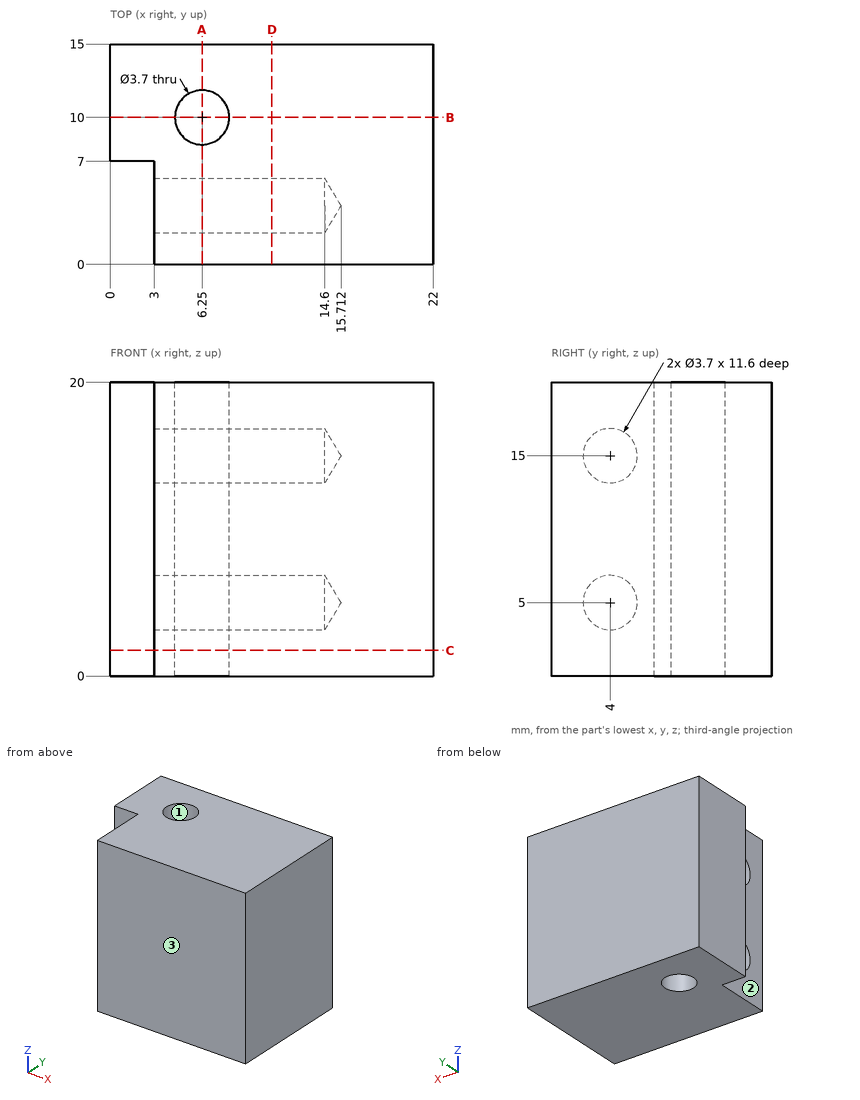
Job drawing, mm, ordinate dimensions from the low corner. One solid piece. Round coordinates to 2 decimals unless told otherwise and drop trailing zeros. Loops run counter-clockwise (first coordinate to the right, second up) from the corner with the lowest first, then second, coordinate; pieces in that order, holes last.
Item 1: Cut at D-D, the plane x = 11. Give the cut face in (y, z).
Item 2: Cut at B-B, the plane y = 10. Give the cut face in (x, z).
Item 3: Mould opens along X. For the marked faces 1, 2 and 3 say: +X half, -X half, draft (parallel to the pull), parting line (faces both ways), or undercut.
Item 4: Drill centre lines: line 1 (Z direction, x = 6.5, y = 4); line 2 (Y direction, x = 6.5, z = 15); line 3 (Y direction, x = 7, z = 14.5). Where is each one in solid material? Low to high.
Item 5: Cut at C-C, the plane z = 1.75. Give the cut face in (x, y).
Item 6: Drop flat-ended pins along their axis: P1, Ø4.5, axis at y = 4, z = 15, coming from the -X side; P2, Ø1.5, axis at x = 1, z = 10, coming from the -Y side. Give the stop position or say it passes through.
Item 7: Cut at A-A, the plane x = 6.25. Give the cut face in (y, z).
A:
1. outline: (0, 0) - (15, 0) - (15, 20) - (0, 20) - close; hole circle Ø3.7 at (4, 5); hole circle Ø3.7 at (4, 15)
2. outline: (0, 0) - (4.4, 0) - (4.4, 20) - (0, 20) - close; (8.1, 0) - (22, 0) - (22, 20) - (8.1, 20) - close
3. face 1: undercut
3. face 2: -X half
3. face 3: draft
4. line 1: z = 0 to 3.15, 6.85 to 13.15, 16.85 to 20
4. line 2: y = 0 to 2.15, 5.85 to 8.17, 11.83 to 15
4. line 3: y = 0 to 2.22, 5.78 to 8.31, 11.69 to 15
5. outline: (0, 7) - (3, 7) - (3, 0) - (22, 0) - (22, 15) - (0, 15) - close; hole circle Ø3.7 at (6.25, 10)
6. P1: stops at x = 3
6. P2: stops at y = 7
7. outline: (0, 0) - (8.15, 0) - (8.15, 20) - (0, 20) - close; (11.85, 0) - (15, 0) - (15, 20) - (11.85, 20) - close; hole circle Ø3.7 at (4, 5); hole circle Ø3.7 at (4, 15)
